The model under review builds one solid part; all positions refer to its coordinate system, in mm. A direction names the side the tool comes from. Give positions to 0.01 mm unless a question says otherwise; leave off trailing zeros. Loops run counter-clockwise (first coordinate to the right, second up) from the corner with the lowest first, then second, coordinate; pieces in that order, holes last. Notation, with made-up numbers: (35.25, 38) - (51.25, 38) arc R26 cw to (51.25, 74) - close; hole circle Ø8 at (71.5, -34). An arc over 180 degrees is marked (long way). Answer as a JSON object with one key per item and string values.
Autodesk Inventor part; units mm, degrees
ref_plane "YZ Plane" through (0, 0, 0) normal (1, 0, 0) x (0, 1, 0)
ref_plane "XZ Plane" through (0, 0, 0) normal (0, 1, 0) x (-1, 0, 0)
ref_plane "XY Plane" through (0, 0, 0) normal (0, 0, 1) x (1, 0, 0)
sketch "Esquisse1" plane through (0, 0, 0) normal (0, 1, 0) x (-1, 0, 0)
  circle A0 centre (0, 0) radius 15
  dimension "d0" = 30
extrude "Extrusion1" add sketch "Esquisse1" along normal blind 150
sketch "Esquisse2" plane through (0, 0, 0) normal (0, 1, 0) x (-1, 0, 0)
  circle A0 centre (0, 0) radius 10
  dimension "d5" = 20
extrude "Extrusion2" add sketch "Esquisse2" along normal blind 154 and the other way blind 5
thread "Filetage2"
chamfer "Chanfrein1" distance 5 angle 45 1 edges at (15, 150, 0)
chamfer "Chanfrein2" distance 5 angle 45 1 edges at (15, 0, 0)
sketch "Esquisse5" plane through (0, -5, 0) normal (0, -1, 0) x (1, 0, 0)
  circle A0 centre (0, 0) radius 12
  dimension "d24" = 24
extrude "Extrusion4" add sketch "Esquisse5" along normal blind 5 and the other way blind 5
sketch "Esquisse3" plane through (0, 0, 0) normal (0, 1, 0) x (-1, 0, 0)
  circle A0 centre (0, 0) radius 10
  circle A1 centre (0, 0) radius 5
  dimension "d33" = 10
extrude "Extrusion3" cut sketch "Esquisse3" along normal blind 154 and the other way blind 72 contours A1
thread "Filetage5"
properties part number "Manche interm"
Q1. Clearance check with flat-ended pins moving along their axes: pin 1 Ø12 at (x, z) = (-3, -1.5) entering from +Y; pin 2 Ø3 at (x, z) = (3, -12) entering from +Y; pin 3 Ø4 at (y, z) = (8, 8.5) entering from +X; pin 4 Ø5 at (x, y) = (11.5, 62.5) entering from +Z. State where each tip first meets the part, or that it passes through.
Results:
{"pin 1": "stops at y = 154", "pin 2": "stops at y = 149.13", "pin 3": "stops at x = 13.52", "pin 4": "stops at z = 12"}
Q2. To check wall thickness, follow probe 1 along Z at (x, y) = (-0.25, 126); probe 2 along Z at (x, y) = (0.75, 43.5); probe 3 along X at (y, z) = (130.5, -2.75). State the ranges of each line that lie inside material, in increasing order. Write a range as [from, to].
Results:
{"probe 1": "z = [-15, -4.99], [4.99, 15]", "probe 2": "z = [-14.98, -4.94], [4.94, 14.98]", "probe 3": "x = [-14.75, -4.18], [4.18, 14.75]"}
Q3. Consider section C-C, the plane y = 7. State the section outline as (x, z) points, plus the area to 3 significant figures.
Results:
{"outline": "circle Ø30 at (0, 0); hole circle Ø10 at (0, 0)", "area": "628 mm^2"}
Q4. For faces 1 (the face through (2.17, 151.97, 9.76)), 2 (the face through (14.985, 74.02, -0.66)), 3 (the face through (-5, 0, 9)), list the 3-axis set-ups (+Z, -Z, +X, -X, +Y, -Y) from which the entire face can be reached by the end or side of a thin tool; tool diameter is ignored.
Results:
{"face 1": "+Y", "face 2": "+Y, -Y", "face 3": "none"}
Q5. The part is to be moulded in two halves that separate along Y. For faces 4 (the face through (-11.99, -5.07, 0.53)), 5 (the face through (2.236, 0.313, -10.068)), 6 (the face through (5.2, -10, 0.2)), say which applies: +Y half, -Y half, draft (parallel to the pull), parting line (faces both ways), or undercut.
Results:
{"face 4": "draft", "face 5": "undercut", "face 6": "-Y half"}
